The listing builds one solid part. Answer for the finished solid, in the listing's coordinates (mm). A direction names the side the tool comes from. Round coordinates to 2 decimals unless told otherwise and drop trailing zeros. Loops run counter-clockwise (first coordinate to the right, second up) from the corner with the lowest first, then second, coordinate; pieces in that order, holes last. Notation, with made-up numbers: (18.5, 28) - (60.5, 28) arc R27 cw to (60.5, 51) - close; hole circle Ø1 at (-5.5, -12). An arc over 180 degrees is marked (long way). One line per item, written item: value.
Autodesk Inventor part; units mm, degrees
ref_plane "YZ Plane" through (0, 0, 0) normal (1, 0, 0) x (0, 1, 0)
ref_plane "XZ Plane" through (0, 0, 0) normal (0, 1, 0) x (-1, 0, 0)
ref_plane "XY Plane" through (0, 0, 0) normal (0, 0, 1) x (1, 0, 0)
sketch "Sketch1" plane through (0, 0, 0) normal (0, 0, 1) x (1, 0, 0)
  line L0 (0, 0) -> (38, 0)
  line L1 (38, 0) -> (38, 40)
  line L2 (38, 40) -> (0, 40)
  line L3 (0, 40) -> (0, 0)
  dimension "d0" = 38
  dimension "d1" = 40
extrude "Extrusion1" add sketch "Sketch1" along normal blind 3
sketch "Sketch2" plane through (0, 0, 3) normal (0, 0, 1) x (1, 0, 0)
  line L0 (38, 0) -> (38, 40)
  line L1 (38, 40) -> (38, 0)
  line L2 (38, 0) -> (34.9318, 0)
  line L3 (35, 37) -> (3, 37)
  line L4 (3, 37) -> (3, 0)
  line L5 (0, 40) -> (0, 0)
  line L6 (0, 0) -> (0, 40)
  line L7 (38, 40) -> (0, 40)
  line L8 (0, 40) -> (38, 40)
  line L9 (35, 37) -> (35, 0)
  line L10 (3, 0) -> (0, 0)
  dimension "d4" = 3
  dimension "d5" = 3
  dimension "d6" = 3
extrude "Extrusion2" add sketch "Sketch2" along normal blind 20
sketch "Sketch3" plane through (38, 0, 0) normal (1, 0, 0) x (0, 0, -1)
  line L0 (-23, 0) -> (-23, 40)
  line L1 (0, 0) -> (-23, 0)
  line L2 (-23, 0) -> (-23, 40)
  line L3 (-23, 40) -> (0, 40)
  line L4 (0, 40) -> (0, 0)
extrude "Extrusion3" add sketch "Sketch3" along normal blind 1.4
sketch "Sketch4" plane through (35, 0, 3) normal (-1, 0, 0) x (0, 0, 1)
  line L0 (0, 37) -> (20, 37)
  line L1 (0, 0) -> (20, 0)
  line L2 (20, 37) -> (0, 37)
  line L3 (0, 37) -> (0, 0)
  line L4 (0, 0) -> (20, 0)
  line L5 (20, 0) -> (20, 37)
  point P0 (-3, 0)
extrude "Extrusion4" cut sketch "Sketch4" against normal blind 1.4
sketch "Sketch5" plane through (0, 0, 0) normal (-1, 0, 0) x (0, 0, 1)
  line L0 (0, 40) -> (23, 40)
  line L1 (23, 40) -> (0, 40)
  line L2 (0, 40) -> (0, 0)
  line L3 (0, 0) -> (23, 0)
  line L4 (23, 0) -> (23, 40)
extrude "Extrusion5" add sketch "Sketch5" along normal blind 1.4
sketch "Sketch6" plane through (3, 0, 3) normal (1, 0, 0) x (0, 0, -1)
  line L0 (0, 37) -> (0, 0)
  line L1 (-20, 0) -> (-20, 37)
  line L2 (0, 37) -> (-20, 37)
  line L3 (-20, 37) -> (-20, 0)
  line L4 (-20, 0) -> (0, 0)
  line L5 (0, 0) -> (0, 37)
  point P0 (3, 0)
extrude "Extrusion6" cut sketch "Sketch6" against normal blind 1.4
sketch "Sketch7" plane through (39.4, 0, 0) normal (0, -1, 0) x (1, 0, 0)
  line L0 (-3, 3) -> (-3, 23)
  line L1 (-3, 4) -> (-5, 4)
  line L2 (-5, 4) -> (-5, 5)
  line L3 (-5, 5) -> (-3, 5)
  line L4 (-3, 5) -> (-3, 4)
  line L5 (-37.8, 3) -> (-3, 3)
  point P0 (-39.4, 0)
  dimension "d17" = 2
  dimension "d18" = 1
  dimension "d19" = 1
extrude "Extrusion7" add sketch "Sketch7" against normal blind 37.0078
sketch "Sketch9" plane through (39.4, 0, 0) normal (0, -1, 0) x (1, 0, 0)
  line L0 (-37.8, 3) -> (-37.8, 23)
  line L1 (-37.8, 4) -> (-35.8, 4)
  line L2 (-35.8, 4) -> (-35.8, 5)
  line L3 (-35.8, 5) -> (-37.8, 5)
  line L4 (-37.8, 5) -> (-37.8, 4)
  line L5 (-37.8, 3) -> (-3, 3)
  point P0 (-39.4, 0)
  dimension "d22" = 2
  dimension "d23" = 1
  dimension "d24" = 1
extrude "Extrusion8" add sketch "Sketch9" against normal blind 37.0078
sketch "Sketch10" plane through (1.6, 37, 3) normal (0, -1, 0) x (1, 0, 0)
  line L0 (0, 2) -> (2, 2)
  line L1 (32.8, 1) -> (32.8, 2)
  line L2 (2, 2) -> (32.8, 2)
  line L3 (32.8, 2) -> (32.8, 1)
  line L4 (32.8, 1) -> (2, 1)
  line L5 (2, 1) -> (2, 2)
  point P0 (-1.6, -3)
extrude "Extrusion9" add sketch "Sketch10" along normal blind 2
sketch "Sketch11" plane through (1.6, 0, 3) normal (1, 0, 0) x (0, 0, -1)
  line L0 (-1, 37) -> (0, 37)
  line L1 (0, 0) -> (-1, 0)
  line L2 (0, 37) -> (-1, 37)
  line L3 (-1, 37) -> (-1, 0)
  line L4 (-1, 0) -> (0, 0)
  line L5 (0, 0) -> (0, 37)
  point P0 (3, 0)
extrude "Extrusion10" add sketch "Sketch11" along normal blind 1
sketch "Sketch12" plane through (36.4, 0, 3) normal (-1, 0, 0) x (0, 0, 1)
  line L0 (0, 0) -> (0, 37)
  line L1 (1, 0) -> (0, 0)
  line L2 (0, 37) -> (1, 37)
  line L3 (1, 37) -> (1, 0)
  line L4 (1, 0) -> (0, 0)
  line L5 (0, 0) -> (0, 37)
  point P0 (-3, 0)
extrude "Extrusion11" add sketch "Sketch12" along normal blind 1
sketch "Sketch13" plane through (39.4, 0, 0) normal (0, -1, 0) x (1, 0, 0)
  line L0 (-4, 3) -> (-36.8, 3)
  line L1 (-33.371, 3) -> (-24.171, 3)
  line L2 (-24.171, 3) -> (-24.171, 1.25)
  line L3 (-24.171, 1.25) -> (-33.371, 1.25)
  line L4 (-33.371, 1.25) -> (-33.371, 3)
  line L5 (-16.671, 3) -> (-7.471, 3)
  line L6 (-7.471, 3) -> (-7.471, 1.25)
  line L7 (-7.471, 1.25) -> (-16.671, 1.25)
  line L8 (-16.671, 1.25) -> (-16.671, 3)
  point P0 (-39.4, 0)
  dimension "d33" = 9.2
  dimension "d34" = 9.2
  dimension "d35" = 7.5
  dimension "d36" = 3.429
  dimension "d37" = 1.75
extrude "Extrusion12" cut sketch "Sketch13" against normal blind 12
sketch "Sketch14" plane through (0, 0, 0) normal (0, 0, -1) x (-1, 0, 0)
  circle A0 centre (-3.68, 12) radius 2.54
  circle A1 centre (-19, 23.43) radius 2.54
  circle A2 centre (-3.68, 34.92) radius 2.54
  circle A3 centre (-34.32, 12) radius 2.54
  circle A4 centre (-34.32, 34.92) radius 2.54
  line L0 (1.4, 0) -> (-39.4, 0)
  line L1 (1.4, 40) -> (1.4, 0)
  line L2 (-39.4, 0) -> (-39.4, 40)
  line L3 (1.4, 40) -> (-39.4, 40)
  point P0 (0, 0)
  dimension "d40" = 5.08
  dimension "d41" = 5.08
  dimension "d42" = 5.08
  dimension "d43" = 5.08
  dimension "d44" = 5.08
  dimension "d45" = 12
  dimension "d46" = 12
  dimension "d47" = 5.08
  dimension "d48" = 5.08
  dimension "d49" = 5.08
  dimension "d50" = 5.08
  dimension "d51" = 5.08
  dimension "d52" = 5.08
  dimension "d53" = 11.43
extrude "Extrusion13" add sketch "Sketch14" along normal blind 12 contours A0 | A1 | A2 | A3 | A4
thread "Thread1"
thread "Thread2"
thread "Thread3"
thread "Thread4"
thread "Thread5"
properties part number "ecog_casing_1"
1) Consider L1, parallel to X at y = 27, z = 17; L2, parallel to X at y = 8, z = 1.5; L3, parallel to X at y = 30, z = 3.5. Determine where each line is inside the solid, lowest interval first.
Final values:
L1: -1.4 to 1.6, 36.4 to 39.4
L2: -1.4 to 6.03, 15.23 to 22.73, 31.93 to 39.4
L3: -1.4 to 2.6, 35.4 to 39.4
2) A cutting plane is placed at C-C on x = 19. Give the vertices of the cut face in (y, z).
Final values:
outline: (0, 0) - (20.89, 0) - (20.89, -12) - (25.97, -12) - (25.97, 0) - (40, 0) - (40, 23) - (37, 23) - (37, 5) - (35, 5) - (35, 4) - (37, 4) - (37, 3) - (0, 3) - close
3) A cutting plane is placed at D-D on y = 7.5. Give the vertices of the cut face in (x, z), and give its area (3 significant figures).
Final values:
outline: (-1.4, 0) - (39.4, 0) - (39.4, 23) - (36.4, 23) - (36.4, 5) - (34.4, 5) - (34.4, 4) - (35.4, 4) - (35.4, 3) - (31.93, 3) - (31.93, 1.25) - (22.73, 1.25) - (22.73, 3) - (15.23, 3) - (15.23, 1.25) - (6.03, 1.25) - (6.03, 3) - (2.6, 3) - (2.6, 4) - (3.6, 4) - (3.6, 5) - (1.6, 5) - (1.6, 23) - (-1.4, 23) - close
area: 216 mm2
4) Each of these flat-tipped pins is pushed along its axis until it touches: pin 1 Ø1.5 at (x, y) = (11, 29) entering from +Z; pin 2 Ø5 at (x, y) = (12, 11) entering from -Z; pin 3 Ø1.1 at (x, z) = (16, 4.5) entering from -Y. Where does it stop, or does it pass through?
Final values:
pin 1: z = 3
pin 2: z = 0
pin 3: y = 35
5) A cutting plane is placed at B-B on x = 26. Give the vertices of the cut face in (y, z).
Final values:
outline: (0, 0) - (40, 0) - (40, 23) - (37, 23) - (37, 5) - (35, 5) - (35, 4) - (37, 4) - (37, 3) - (12, 3) - (12, 1.25) - (0, 1.25) - close
6) A cutting plane is placed at A-A on y = 30. Give the vertices of the cut face in (x, z).
Final values:
outline: (-1.4, 0) - (39.4, 0) - (39.4, 23) - (36.4, 23) - (36.4, 5) - (34.4, 5) - (34.4, 4) - (35.4, 4) - (35.4, 3) - (2.6, 3) - (2.6, 4) - (3.6, 4) - (3.6, 5) - (1.6, 5) - (1.6, 23) - (-1.4, 23) - close
7) For faces 4 (the cylindrical face through (4, 32.4, -5.9)), 5 (the flat face through (22.729, 6, 2)), 6 (the flat face through (19, 23, 3)), 7 (the flat face through (21, 0, 2)), determine the directions among +Z, -Z, +X, -X, +Y, -Y from which every point of the face is accessible in a straight line to the end or side of a thin tool.
Final values:
face 4: -Z
face 5: +Z, -Y
face 6: -Y
face 7: +Z, -Z, +X, -X, -Y
8) For a pull along Y with two mould halves and no side action, classify faces 1 (the flat face through (36.4, 19, 14)), 2 (the flat face through (19, 40, 11)), 3 (the cylindrical face through (31.974, 12.973, -5.916)) as released by +Y, released by -Y, zero draft, split by the parting line, or undercut.
Final values:
face 1: zero draft
face 2: released by +Y
face 3: undercut
